Source: CAD feature listing. Evaluate the final solid. Frame: model axes, mm. A direction names the side the tool comes from. Round coordinates to 2 decimals unless told otherwise and drop trailing zeros. Loops run counter-clockwise (first coordinate to the right, second up) from the corner with the lowest first, then second, coordinate; pieces in that order, holes last.
Item 1: Section query A-A on x = 16.25. Return loops of the section in (y, z).
Item 2: First-contact query: P1, Ø4, axis at y = -15, z = 13, coming from the +X side; P2, Ø10, axis at y = -26.5, z = 24, coming from the -X side; P3, Ø6, axis at x = 20, y = -52, coming from the -Z side; P4, Ø1.5, axis at x = 24.5, z = 12, coming from the +Y side. Flat tips, straight axial feed; report the tip coordinate or a pass-through.
Item 3: Section query B-B on z = 21.5. Return loops of the section in (x, y), then the cut area to 3 significant figures.
Item 4: Section query D-D on x = 29.5. Return loops of the section in (y, z).
Item 5: Pull-direction query (X, two-part tool) for faces 1 (the cylindrical face through (18.557, -50.483, 5.864)), 2 (the flat face through (16, -48.8, 19)), 3 (the flat face through (16, 0, 16)); classes: released by +X, released by -X, zero draft, split by the parting line, or undercut.
Item 6: Access query for faces 4 (the flat face through (16, -49.3, 16)), 5 (the flat face through (16, -54.3, 11)), 6 (the flat face through (16, -58.2, 10)). Directions: +Z, -Z, +X, -X, +Y, -Y. A direction counts if a zero-diameter tool reaches every point of the face in a straight line with its end or side. Return the directions, or none.
Item 7: Ray query, L1, parallel to Z at x = 16, y = -49; L2, parallel to X at y = -49, z = 16; L3, parallel to Y at x = 8.5, z = 11. Return the intervals inside material, ascending.
Item 8: Section query C-C on y = -38. Return loops of the section in (x, z), then the cut area to 3 significant figures.
```python
from build123d import *

# Parameters (mm, degrees)
SKETCH001_R  = 16.25
PAD001_DEPTH = 49.3
SKETCH002_R  = 11.408958
POCKET_DEPTH = 0.5
SKETCH003_R  = 6.29816
PAD002_DEPTH = 0.5
SKETCH004_R  = 5
PAD003_DEPTH = 2.4
SKETCH005_R  = 2
PAD004_DEPTH = 2.6
PAD005_DEPTH = 3.9


with BuildPart() as part:
    # Sketch001 → Pad001 (new body)
    with BuildSketch(Plane.XZ):
        with Locations((16.25, 16.25)):
            Circle(SKETCH001_R)
    extrude(amount=PAD001_DEPTH)

    # Sketch002 (on Face3 of Pad001) → Pocket (cut)
    with BuildSketch(Plane.XZ.offset(49.3)):
        with Locations((16.25, 16.25)):
            Circle(SKETCH002_R)
    extrude(amount=-POCKET_DEPTH, mode=Mode.SUBTRACT)

    # Sketch003 (on Face5 of Pocket) → Pad002 (join)
    with BuildSketch(Plane.XZ.offset(48.8)):
        with Locations((16.25, 10.3)):
            Circle(SKETCH003_R)
    extrude(amount=PAD002_DEPTH)

    # Sketch004 (on Face9 of Pad002) → Pad003 (join)
    with BuildSketch(Plane.XZ.offset(49.3)):
        with Locations((16.25, 10.3)):
            Circle(SKETCH004_R)
    extrude(amount=PAD003_DEPTH)

    # Sketch005 (on Face12 of Pad003) → Pad004 (join)
    with BuildSketch(Plane.XZ.offset(51.7)):
        with Locations((16.25, 10.3)):
            Circle(SKETCH005_R)
    extrude(amount=PAD004_DEPTH)

    # Sketch006 (on Face14 of Pad004) → Pad005 (join)
    with BuildSketch(Plane.XZ.offset(54.3)):
        with BuildLine():
            ThreePointArc((14.25, 10.3), (16.25, 8.3), (18.25, 10.3))
            Line((14.25, 10.3), (18.25, 10.3))
        make_face()
    extrude(amount=PAD005_DEPTH)


solid = part.part
```
Data:
1. outline: (-58.2, 8.3) - (-51.7, 8.3) - (-51.7, 5.3) - (-49.3, 5.3) - (-49.3, 0) - (0, 0) - (0, 32.5) - (-49.3, 32.5) - (-49.3, 27.66) - (-48.8, 27.66) - (-48.8, 16.6) - (-49.3, 16.6) - (-49.3, 15.3) - (-51.7, 15.3) - (-51.7, 12.3) - (-54.3, 12.3) - (-54.3, 10.3) - (-58.2, 10.3) - close
2. P1: stops at x = 32.45
2. P2: stops at x = 0.23
2. P3: stops at z = 0.18
2. P4: stops at y = 0
3. outline: (0.87, -49.3) - (6.12, -49.3) - (6.12, -48.8) - (26.38, -48.8) - (26.38, -49.3) - (31.63, -49.3) - (31.63, 0) - (0.87, 0) - close
3. area: 1,510 mm2
4. outline: (-49.3, 6.84) - (0, 6.84) - (0, 25.66) - (-49.3, 25.66) - close
5. face 1: split by the parting line
5. face 2: undercut
5. face 3: zero draft
6. face 4: -Y
6. face 5: +Z, +X, -X, -Y
6. face 6: +Z, -Z, +X, -X, -Y
7. L1: z = 0 to 16.59, 27.66 to 32.5
7. L2: x = 0 to 4.84, 13.57 to 18.93, 27.66 to 32.5
7. L3: y = -48.8 to 0
8. outline: circle Ø32.5 at (16.25, 16.25)
8. area: 830 mm2
